CAD build for the part. Positions are in the model's coordinates, mm. Give positions to 0.01 mm unless a question says otherwise; leave off trailing zeros. Order: outer loops, then holes, each group sorted by start corner. A loop starts at its lowest first (then second) coordinate and runs counter-clockwise, first axis right, second up.
```python
from build123d import *

# Parameters (mm, degrees)
SKETCH_1_W      = 110
SKETCH_1_H      = 32
SKETCH_1_R      = 2.1
EXTRUDE_1_DEPTH = 2
FILLET_1_R      = 2


with BuildPart() as part:
    # ｽｹｯﾁ1 → ﾎﾞｽ - 押し出し1 (new body)
    with BuildSketch(Plane.XY):
        Rectangle(SKETCH_1_W, SKETCH_1_H)
        with Locations((31, 0)):
            Circle(SKETCH_1_R, mode=Mode.SUBTRACT)
        with Locations(Location((-31, 0, 0), (0, 0, 180))):
            Circle(SKETCH_1_R, mode=Mode.SUBTRACT)
        with Locations((50, 11)):
            Circle(SKETCH_1_R, mode=Mode.SUBTRACT)
        with Locations(Location((-50, 11, 0), (0, 0, 180))):
            Circle(SKETCH_1_R, mode=Mode.SUBTRACT)
        with Locations((-50, -11)):
            Circle(SKETCH_1_R, mode=Mode.SUBTRACT)
        with Locations(Location((50, -11, 0), (0, 0, 180))):
            Circle(SKETCH_1_R, mode=Mode.SUBTRACT)
    extrude(amount=EXTRUDE_1_DEPTH)

    # ﾌｨﾚｯﾄ1
    fillet_1_edges = [part.edges().sort_by_distance(p)[0] for p in [
        (55, -16, 1),
        (-55, -16, 1),
        (-55, 16, 1),
        (55, 16, 1),
    ]]
    fillet(fillet_1_edges, radius=FILLET_1_R)


solid = part.part
```
Item 1: Drop a flat-ended pin along its axis: pin 1 Ø2 at (x, y) = (-14, 3.5) entering from -Z. Give the stop position or say it passes through.
Item 2: Slice it at C-C (y = -11). Give the cut face in (x, z), and give its area (3 significant figures).
Item 3: Two-plate mould, pull along X, no slides. Class faces 1 (the face through (-47.997, -10.369, 0.986)), 2 (the face through (-28.9, -0.09, 0.99)), 3 (the face through (-1, 16, 1)), 4 (the face through (54.4, 15.43, 1.01)): released by +X, released by -X, zero draft, split by the parting line, or undercut.
Item 4: Slice it at D-D (z = 0.6). Give the cut face in (x, y).
Item 5: Slice it at A-A (x = 31). Give the cut face in (y, z), and give its area (3 significant figures).
Item 6: Slice it at B-B (x = -50). Give the cut face in (y, z).
Item 7: Wall check: L1, parallel to Y at x = 50, z = 1.05; L2, parallel to Y at x = 31, z = 0.4; L3, parallel to X at y = -1, z = 0.2. Give the ranges that are in metal, low to high.
A:
1. pin 1: stops at z = 0
2. outline: (-55, 0) - (-52.1, 0) - (-52.1, 2) - (-55, 2) - close; (-47.9, 0) - (47.9, 0) - (47.9, 2) - (-47.9, 2) - close; (52.1, 0) - (55, 0) - (55, 2) - (52.1, 2) - close
2. area: 203 mm2
3. face 1: undercut
3. face 2: undercut
3. face 3: zero draft
3. face 4: released by +X
4. outline: (-55, -14) arc R2 ccw to (-53, -16) - (53, -16) arc R2 ccw to (55, -14) - (55, 14) arc R2 ccw to (53, 16) - (-53, 16) arc R2 ccw to (-55, 14) - close; hole circle Ø4.2 at (-50, -11); hole circle Ø4.2 at (-50, 11); hole circle Ø4.2 at (-31, 0); hole circle Ø4.2 at (31, 0); hole circle Ø4.2 at (50, -11); hole circle Ø4.2 at (50, 11)
5. outline: (-16, 0) - (-2.1, 0) - (-2.1, 2) - (-16, 2) - close; (2.1, 0) - (16, 0) - (16, 2) - (2.1, 2) - close
5. area: 55.6 mm2
6. outline: (-16, 0) - (-13.1, 0) - (-13.1, 2) - (-16, 2) - close; (-8.9, 0) - (8.9, 0) - (8.9, 2) - (-8.9, 2) - close; (13.1, 0) - (16, 0) - (16, 2) - (13.1, 2) - close
7. L1: y = -16 to -13.1, -8.9 to 8.9, 13.1 to 16
7. L2: y = -16 to -2.1, 2.1 to 16
7. L3: x = -55 to -32.85, -29.15 to 29.15, 32.85 to 55
